from build123d import *

# Parameters (mm, degrees)
SKETCH1_R                = 24.5
SKETCH1_R_2              = 22.5
BOSS_EXTRUDE1_DEPTH      = 10
BOSS_EXTRUDE1_DEPTH_BACK = 15
SKETCH2_R                = 22.735866394
BOSS_EXTRUDE2_DEPTH      = 2
BOSS_EXTRUDE3_DEPTH      = 2
SKETCH4_R                = 28.5
SKETCH4_R_2              = 24.5
BOSS_EXTRUDE4_DEPTH      = 3


with BuildPart() as part:
    # Sketch1 → Boss-Extrude1 (new body, two sides)
    with BuildSketch(Plane.XY) as boss_extrude1_sk:
        with Locations((-8.522732981, 9.177701176)):
            Circle(SKETCH1_R)
        with Locations((-8.522732981, 9.177701176)):
            Circle(SKETCH1_R_2, mode=Mode.SUBTRACT)
    extrude(amount=BOSS_EXTRUDE1_DEPTH)
    extrude(boss_extrude1_sk.sketch, amount=-BOSS_EXTRUDE1_DEPTH_BACK)

    # Sketch2 → Boss-Extrude2 (add)
    with BuildSketch(Plane.XY.offset(10)):
        with Locations((-8.522732981, 9.177701176)):
            Circle(SKETCH2_R)
    extrude(amount=-BOSS_EXTRUDE2_DEPTH)

    # Sketch3 → Boss-Extrude3 (add)
    with BuildSketch(Plane(origin=(0, 0, -15), x_dir=(-1, 0, 0), z_dir=(0, 0, -1))):
        with BuildLine():
            Line((30.460143949, 14.177701176), (17.182987019, 14.177701176))
            ThreePointArc((17.182987019, 14.177701176), (18.181991244, 11.765891627), (18.522732981, 9.177701176))
            ThreePointArc((18.522732981, 9.177701176), (18.181991244, 6.589510725), (17.182987019, 4.177701176))
            Line((17.182987019, 4.177701176), (30.460143949, 4.177701176))
            ThreePointArc((30.460143949, 4.177701176), (30.881643361, 6.661925629), (31.022732981, 9.177701176))
            ThreePointArc((31.022732981, 9.177701176), (30.881643361, 11.693476723), (30.460143949, 14.177701176))
        make_face()
        with BuildLine():
            Line((17.182987019, 14.177701176), (16.522732981, 14.177701176))
            Line((16.522732981, 14.177701176), (16.522732981, 4.177701176))
            Line((16.522732981, 4.177701176), (17.182987019, 4.177701176))
            ThreePointArc((17.182987019, 4.177701176), (18.181991244, 6.589510725), (18.522732981, 9.177701176))
            ThreePointArc((18.522732981, 9.177701176), (18.181991244, 11.765891627), (17.182987019, 14.177701176))
        make_face()
        with BuildLine():
            Line((16.522732981, 4.177701176), (16.522732981, 14.177701176))
            Line((16.522732981, 14.177701176), (17.182987019, 14.177701176))
            ThreePointArc((17.182987019, 14.177701176), (8.522732981, 19.177701176), (-0.137521057, 14.177701176))
            Line((-0.137521057, 14.177701176), (0.522732981, 14.177701176))
            Line((0.522732981, 14.177701176), (0.522732981, 4.177701176))
            Line((0.522732981, 4.177701176), (-0.137521057, 4.177701176))
            ThreePointArc((-0.137521057, 4.177701176), (8.522732981, -0.822298824), (17.182987019, 4.177701176))
            Line((17.182987019, 4.177701176), (16.522732981, 4.177701176))
        make_face()
        with BuildLine():
            Line((0.522732981, 14.177701176), (-0.137521057, 14.177701176))
            ThreePointArc((-0.137521057, 14.177701176), (-1.477267019, 9.177701176), (-0.137521057, 4.177701176))
            Line((-0.137521057, 4.177701176), (0.522732981, 4.177701176))
            Line((0.522732981, 4.177701176), (0.522732981, 14.177701176))
        make_face()
        with BuildLine():
            ThreePointArc((-0.137521057, 4.177701176), (-1.477267019, 9.177701176), (-0.137521057, 14.177701176))
            Line((-0.137521057, 14.177701176), (-13.414677988, 14.177701176))
            ThreePointArc((-13.414677988, 14.177701176), (-13.836177399, 11.693476723), (-13.977267019, 9.177701176))
            ThreePointArc((-13.977267019, 9.177701176), (-13.836177399, 6.661925629), (-13.414677988, 4.177701176))
            Line((-13.414677988, 4.177701176), (-0.137521057, 4.177701176))
        make_face()
    extrude(amount=-BOSS_EXTRUDE3_DEPTH)

    # Sketch4 → Boss-Extrude4 (add)
    with BuildSketch(Plane(origin=(0, 0, -15), x_dir=(-1, 0, 0), z_dir=(0, 0, -1))):
        with Locations((8.522732981, 9.177701176)):
            Circle(SKETCH4_R)
        with Locations((8.522732981, 9.177701176)):
            Circle(SKETCH4_R_2, mode=Mode.SUBTRACT)
    extrude(amount=-BOSS_EXTRUDE4_DEPTH)


solid = part.part
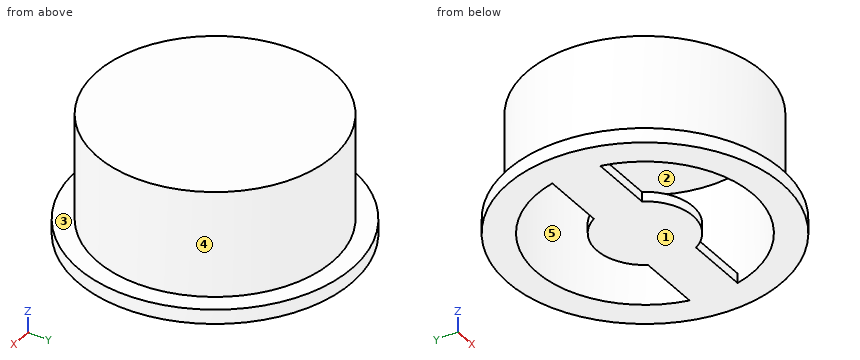
Work out the finished part from the listing and answer in its coordinate system (mm). Face numbers are marked on the shaded views. A direction names the side the tool comes from. Give positions to 0.01 mm unless a question says otherwise; leave off trailing zeros. Loops run counter-clockwise (first coordinate to the right, second up) from the corner with the lowest first, then second, coordinate; pieces in that order, holes last. Notation, with made-up numbers: (52, -35) - (110, -35) arc R28 ccw to (110, -5) - close; hole circle Ø7 at (84.25, 67.5). An arc over 180 degrees is marked (long way). Answer in a Markdown table with one row per item. Add a question column.
Q1. The part is cut by section C-C (y = -6.5). Determine the outline of the cut face in (x, z).
Q2. Consider line 1 along Y through (x, z) = (-8.5, -2.75); line 2 along Z through (x, y) = (12, 7.5); line 3 along Z through (x, y) = (15, -4.5). Determine where each line is inside the solid, lowest interval first.
Q3. Determine the mould class of the marked faces 3, 4 and 5 for opening direction X: released by +X, released by -X, zero draft, split by the parting line, or undercut.
Q4. A tool of negligible diameter and unlimited length cuts with its end or side. For the marked faces 1 and 2, from which of +Z, -Z, +X, -X, +Y, -Y can it reach the whole face along a straight path? Write none if from no direction.
Q5. The part is cut by section A-A (x = -3.5). Determine the outline of the cut face in (y, z), and give its area (3 significant figures).
Q6. Each of these flat-tipped pins is pushed along its axis until it touches: P1, Ø3, axis at y = 28.5, z = 6.5, coming from the +X side; P2, Ø2, axis at x = -6.5, y = -7.5, coming from the -Z side; P3, Ø6, axis at y = -5, z = 1, coming from the -X side. Where does it stop, or does it pass through?
Q7. The part is cut by section D-D (z = 1.5). Determine the outline of the cut face in (x, y).
Q8. The part is cut by section B-B (y = 10.5). Determine the outline of the cut face in (x, z).
Solution:
| question | item | result |
|---|---|---|
| 1 | outline | (-32.32, -15) - (-24.66, -15) - (-24.66, 8) - (7.62, 8) - (7.62, -15) - (15.28, -15) - (15.28, -12) - (10.3, -12) - (10.3, 10) - (-27.35, 10) - (-27.35, -12) - (-32.32, -12) - close |
| 2 | line 1 | y = -15.32 to -13.32, 31.68 to 33.68 |
| 2 | line 2 | z = -15 to -13, 8 to 10 |
| 2 | line 3 | z = -15 to -12 |
| 3 | face 3 | zero draft |
| 3 | face 4 | split by the parting line |
| 3 | face 5 | undercut |
| 4 | face 1 | -Z, +X, -X, +Y, -Y |
| 4 | face 2 | none |
| 5 | outline | (-18.88, -15) - (-12.75, -15) - (-12.75, 8) - (31.11, 8) - (31.11, -15) - (37.23, -15) - (37.23, -12) - (33.16, -12) - (33.16, 10) - (-14.8, 10) - (-14.8, -12) - (-18.88, -12) - close; (0.53, -15) - (17.82, -15) - (17.82, -13) - (0.53, -13) - close |
| 5 | area | 249 mm² |
| 6 | P1 | stops at x = 8.29 |
| 6 | P2 | stops at z = 8 |
| 6 | P3 | stops at x = -30.32 |
| 7 | outline | circle Ø49 at (-8.52, 9.18); hole circle Ø45 at (-8.52, 9.18) |
| 8 | outline | (-36.99, -15) - (19.95, -15) - (19.95, -12) - (15.94, -12) - (15.94, 10) - (-32.99, 10) - (-32.99, -12) - (-36.99, -12) - close; hole (-30.98, -13) - (13.94, -13) - (13.94, 8) - (-30.98, 8) - close |
